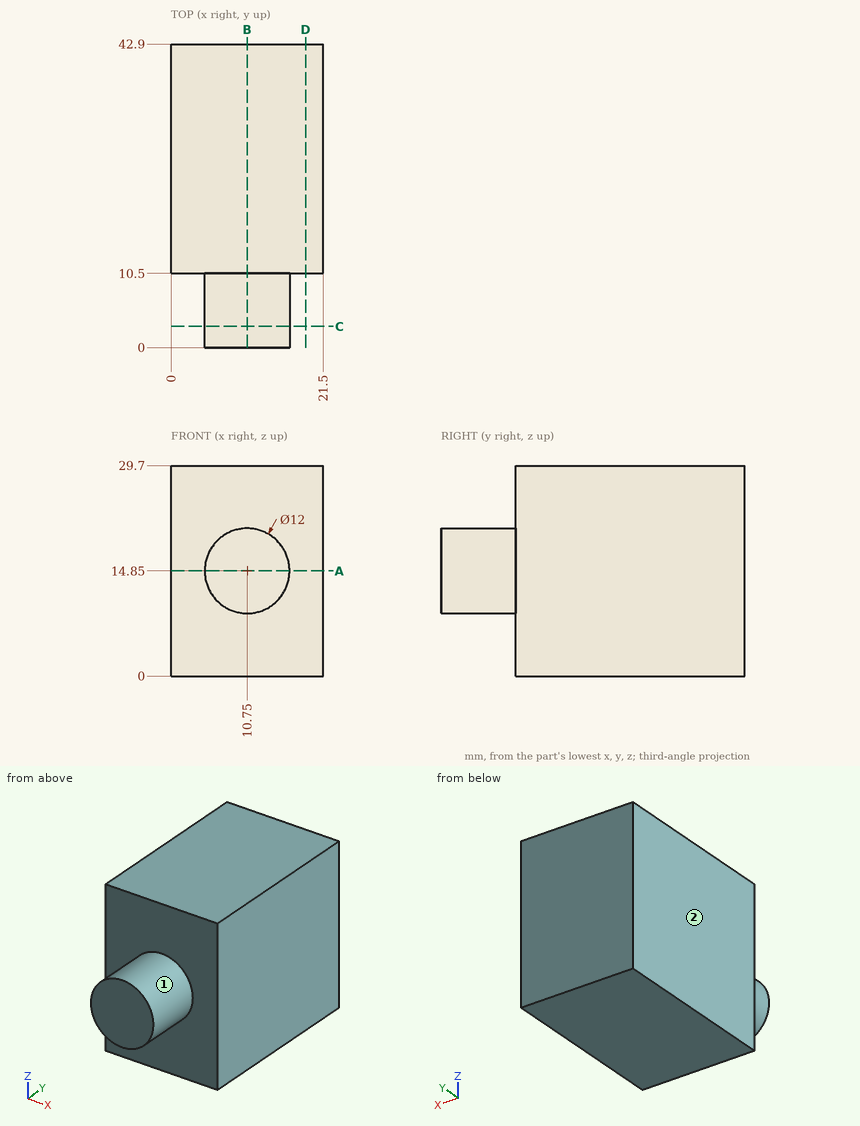
Could you check a few things on this drawing? It's one solid part, dimensions in mm from its lowest x, y, z. A direction names the side the tool comes from. Give positions to 0.01 mm unless a question says otherwise; leave off trailing zeros. Loops run counter-clockwise (first coordinate to the right, second up) from the corner with the lowest first, then second, coordinate; pieces in that order, holes last. Notation, with made-up numbers: (34, 68) -> (75, 68) arc R29 ccw to (75, 92) -> close; hole circle Ø1 at (-16.75, 18.25). An arc over 180 degrees is marked (long way). Use one line per item in the form item = value. Start each with the question number.
1) Imagine slicing it at B-B (x = 10.75). Please give me the cut outline in (y, z), then the cut area to 3 significant figures.
2) Which directions (+Z, -Z, +X, -X, +Y, -Y) give clear straight access to the entire face, cutting with the end or side of a thin tool? Please do the marked faces 1 and 2.
3) Imagine slicing it at D-D (x = 19). Please give me the cut outline in (y, z), then the cut area to 3 significant figures.
4) Imagine slicing it at A-A (z = 14.85). Please give me the cut outline in (x, y).
5) For P1, Ø3, axis at x = 7.5, y = 7, coming from the +Z side, with a flat end and sliding along its axis, tell me the tip position at first contact or that it passes through.
6) Imagine slicing it at C-C (y = 3). Please give me the cut outline in (x, z), then the cut area to 3 significant figures.
7) Please list where these lines run through material, in increasing order: line 1 along Y through (x, z) = (8.5, 1.5); line 2 along Z through (x, y) = (14.5, 8); line 3 along Z through (x, y) = (6, 3).
Check values:
q1.outline = (0, 8.85) -> (10.5, 8.85) -> (10.5, 0) -> (42.9, 0) -> (42.9, 29.7) -> (10.5, 29.7) -> (10.5, 20.85) -> (0, 20.85) -> close
q1.area = 1,090 mm^2
q2.face_1 = -Y
q2.face_2 = +Z, -Z, -X, +Y, -Y
q3.outline = (10.5, 0) -> (42.9, 0) -> (42.9, 29.7) -> (10.5, 29.7) -> close
q3.area = 962 mm^2
q4.outline = (0, 10.5) -> (4.75, 10.5) -> (4.75, 0) -> (16.75, 0) -> (16.75, 10.5) -> (21.5, 10.5) -> (21.5, 42.9) -> (0, 42.9) -> close
q5.P1 = 20.59
q6.outline = circle Ø12 at (10.75, 14.85)
q6.area = 113 mm^2
q7.line_1 = 10.5 to 42.9
q7.line_2 = 10.17 to 19.53
q7.line_3 = 11.18 to 18.52
